Could you check a few things on this model? Use its own coordinates, in mm. A direction names the side the tool comes from. Give positions to 0.01 mm unless a question says otherwise; leave off trailing zeros. Order: outer loops, then holes, each group sorted by start corner. A loop starts at its lowest first (then second) coordinate and runs counter-clockwise, first axis right, second up. Notation, with made-up numbers: (6, 9.5) -> (23, 9.5) arc R29 ccw to (23, 36.5) -> close; hole circle Ø1 at (77.5, 89). An arc over 180 degrees is marked (long way). Answer as CSV lines item,"result". Start each with the question number.
(1) I want a section at D-D (y = 8.25). Please give me the cut outline in (x, z), plus the area to 3 significant figures.
(2) I want a section at B-B (x = 62). Please give me the cut outline in (y, z), plus the area to 3 significant figures.
(3) On a 3-axis mill with a long thin cutter (end or side, diameter ignored), from which of +Z, -Z, +X, -X, +Y, -Y can I reach the whole of each face in a straight line? I mean faces 4 (the face through (-5.734, 12, 4)), 5 (the face through (70.106, 12, 4)), 6 (the face through (63.8, -5, 5)), 7 (the face through (59.714, 12, 4)). Say none if no direction works.
(4) I want a section at C-C (y = 12.25). Please give me the cut outline in (x, z), plus the area to 3 significant figures.
(5) I want a section at A-A (z = 5.75). Please give me the cut outline in (x, y), plus the area to 3 significant figures.
(6) I need wall thicknesses on L1, parallel to X at y = 12.5, z = 4; L2, parallel to Y at x = -6, z = 7; L3, parallel to Z at x = 1.5, y = 10. Which ranges of each line are inside material? Lowest first, please.
(7) We'd pull the mould along X, two halves only. Please class faces 1 (the face through (4.753, 12, 4)), 2 (the face through (65, 12, 2.2)), 3 (the face through (-14.514, -3.97, 7.714)): released by +X, released by -X, zero draft, split by the parting line, or undercut.
(8) Will these pins go through, and if not, where does the flat tip stop? pin 1 Ø3 at (x, z) = (-4.5, 3) entering from -Y; pin 2 Ø1.5 at (x, z) = (69.5, 4) entering from +Y; pin 3 Ø2.5 at (y, z) = (13, 4) entering from +X; pin 4 Ø1 at (x, z) = (33.5, 6.5) entering from +Y.
```python
from build123d import *

# Parameters (mm, degrees)
SKETCH009_W   = 97.773254
SKETCH009_H   = 27.607625
PAD006_DEPTH  = 2
FILLET003_R   = 10
SKETCH010_W   = 1.5
SKETCH010_H   = 4.720073
SKETCH010_H_2 = 4.777608
PAD007_DEPTH  = 2.5
SKETCH011_W   = 10.487562
SKETCH011_H   = 3
SKETCH011_W_2 = 10.392681
PAD008_DEPTH  = 4.5


with BuildPart() as part:
    # Sketch009 → Pad006 (new body)
    with BuildSketch(Plane.XY):
        with Locations((31.520691, 6.826573)):
            Rectangle(SKETCH009_W, SKETCH009_H)
    extrude(amount=PAD006_DEPTH)

    # Fillet003
    fillet003_edges = [part.edges().sort_by_distance(p)[0] for p in [
        (-17.365936, -6.977239, 1),
        (80.407318, -6.977239, 1),
        (80.407318, 20.630386, 1),
        (-17.365936, 20.630386, 1),
    ]]
    fillet(fillet003_edges, radius=FILLET003_R)

    # Sketch010 (on Face2 of Fillet003) → Pad007 (join)
    with BuildSketch(Plane(origin=(0, 0, 0), x_dir=(1, 0, 0), z_dir=(0, 0, -1))):
        with Locations((-0.567265, 4.592866)):
            Rectangle(SKETCH010_W, SKETCH010_H)
        with Locations((64.55027, 4.620095)):
            Rectangle(SKETCH010_W, SKETCH010_H_2)
    extrude(amount=PAD007_DEPTH)

    # Sketch011 (on Face2 of Pad007) → Pad008 (join)
    with BuildSketch(Plane(origin=(0, 0, 0), x_dir=(1, 0, 0), z_dir=(0, 0, -1))):
        with Locations((-0.490359, -12.412728)):
            Rectangle(SKETCH011_W, SKETCH011_H)
        with Locations((64.90986, -12.423971)):
            Rectangle(SKETCH011_W_2, SKETCH011_H)
    extrude(amount=PAD008_DEPTH)


with BuildPart() as part_1:
    # Body004 placement: moved
    add(part.part.moved(Location((0, 0, 6.7))))


solid = part_1.part
```
Final values:
1,outline,"(-17.37, 6.7) -> (80.41, 6.7) -> (80.41, 8.7) -> (-17.37, 8.7) -> close"
1,area,"196 mm²"
2,outline,"(-6.98, 6.7) -> (10.92, 6.7) -> (10.92, 2.2) -> (13.92, 2.2) -> (13.92, 6.7) -> (20.63, 6.7) -> (20.63, 8.7) -> (-6.98, 8.7) -> close"
2,area,"68.7 mm²"
3,face 4,"-Z, -X, +Y, -Y"
3,face 5,"-Z, +X, +Y, -Y"
3,face 6,"-Z, -Y"
3,face 7,"-Z, +Y, -Y"
4,outline,"(-17.23, 6.7) -> (-5.73, 6.7) -> (-5.73, 2.2) -> (4.75, 2.2) -> (4.75, 6.7) -> (59.71, 6.7) -> (59.71, 2.2) -> (70.11, 2.2) -> (70.11, 6.7) -> (80.28, 6.7) -> (80.28, 8.7) -> (-17.23, 8.7) -> close"
4,area,"289 mm²"
5,outline,"(-5.73, 10.91) -> (4.75, 10.91) -> (4.75, 13.91) -> (-5.73, 13.91) -> close; (-1.32, -6.95) -> (0.18, -6.95) -> (0.18, -2.23) -> (-1.32, -2.23) -> close; (59.71, 10.92) -> (70.11, 10.92) -> (70.11, 13.92) -> (59.71, 13.92) -> close; (63.8, -7.01) -> (65.3, -7.01) -> (65.3, -2.23) -> (63.8, -2.23) -> close"
5,area,"76.9 mm²"
6,L1,"-5.73 to 4.75, 59.71 to 70.11"
6,L2,"-6.98 to 20.63"
6,L3,"6.7 to 8.7"
7,face 1,"undercut"
7,face 2,"zero draft"
7,face 3,"released by -X"
8,pin 1,"y = 10.91"
8,pin 2,"y = 13.92"
8,pin 3,"x = 70.11"
8,pin 4,"y = 20.63"
